Geometry: final body of the model. Coordinates: model frame, mm. A direction names the side the tool comes from. Coordinates: 2 decimals unless noted, no trailing zeros. Write each loop counter-clockwise with the first axis right and the second up, starting at its lowest first coordinate (ties: lowest second). Pieces come first, ordered by that corner, then holes. Notation, with made-up numbers: (74, -36) -> (111, -36) arc R28 cw to (111, -1) -> close; hole circle Ø9 at (24, -37.5). An arc over 180 degrees is marked (long way). One line per item, written item: value. Start each with the question number.
from build123d import *

# Parameters (mm, degrees)
SKETCH1_R               = 40
BOSS_EXTRUDE1_DEPTH     = 100
CUT_EXTRUDE1_DEPTH      = 41
CUT_EXTRUDE1_DEPTH_BACK = 41


with BuildPart() as part:
    # Sketch1 → Boss-Extrude1 (new body)
    with BuildSketch(Plane(origin=(0, 0, 0), x_dir=(1, 0, 0), z_dir=(0, 1, 0))):
        Circle(SKETCH1_R)
        Polygon((0, -20), (-20, 0), (0, 20), (20, 0), align=None, mode=Mode.SUBTRACT)
    extrude(amount=BOSS_EXTRUDE1_DEPTH)

    # Sketch2 → Cut-Extrude1 (cut, two sides)
    with BuildSketch(Plane.XY) as cut_extrude1_sk:
        Polygon((-40, 20), (40, 100), (-40, 100), align=None)
    extrude(amount=CUT_EXTRUDE1_DEPTH, mode=Mode.SUBTRACT)
    extrude(cut_extrude1_sk.sketch, amount=-CUT_EXTRUDE1_DEPTH_BACK, mode=Mode.SUBTRACT)


solid = part.part
Q1. Cut plane B-B on x = -9. Output: boundary loops of the cut face in (y, z), and give its area (3 significant figures).
Q2. Cut plane D-D on z = 24. Output: boundary loops of the cut face in (x, y).
Q3. Cut plane C-C on y = 37. Output: boundary loops of the cut face in (x, z).
Q4. Cut plane A-A on z = 1.5. Output: boundary loops of the cut face in (x, y).
Q5. Access query for faces 1 (the flat face through (10, 31, -10)), 2 (the flat face through (8, 0, 17)). Directions: +Z, -Z, +X, -X, +Y, -Y. A direction counts if a zero-diameter tool reaches every point of the face in a straight line with its end or side. Return the directions, or none.
Q6. Draft query along Z for faces 3 (the cylindrical face through (36.95, 38.19, 15.32)), 4 (the flat face through (8, 68, 17)), 5 (the flat face through (-10, 23, -10)). Return one class per face: pulls with the +Z half, pulls with the -Z half, needs draft (parallel to the pull), parting line crosses it, or undercut.
Q7. Line query: L1, parallel to X at y = 19.5, z = 16; L2, parallel to Z at x = 12, y = 17; L3, parallel to Z at x = 11, y = 39.5. Output: solid intervals per line, ascending. Write a range as from..to.
Q8. First-contact query: P1, Ø10, axis at x = 29, y = 43, coming from the -Z side; P2, Ø8, axis at y = 60, z = -1, coming from the -X side; P3, Ø1.5, axis at x = 24, y = 74.5, coming from the -Z side. Flat tips, straight axial feed; report the tip coordinate or a pass-through.
Solution:
1. outline: (0, -38.97) -> (51, -38.97) -> (51, -11) -> (0, -11) -> close; (0, 11) -> (51, 11) -> (51, 38.97) -> (0, 38.97) -> close
1. area: 2,850 mm²
2. outline: (-32, 0) -> (32, 0) -> (32, 92) -> (-32, 28) -> close
3. outline: (-23, -32.73) arc R40 ccw (long way) to (-23, 32.73) -> close; hole (-20, 0) -> (0, -20) -> (20, 0) -> (0, 20) -> close
4. outline: (-39.97, 0) -> (-18.5, 0) -> (-18.5, 41.5) -> (-39.97, 20.03) -> close; (18.5, 0) -> (39.97, 0) -> (39.97, 99.97) -> (18.5, 78.5) -> close
5. face 1: +Y, -Y
5. face 2: +Z, -Z, +X, -X, -Y
6. face 3: parting line crosses it
6. face 4: needs draft
6. face 5: undercut
7. L1: -36.66..-4, 4..36.66
7. L2: -38.16..-8, 8..38.16
7. L3: -38.46..-9, 9..38.46
8. P1: z = -32
8. P2: x = 15
8. P3: z = -32.55
